from build123d import *

# Parameters (mm, degrees)
SKETCH1_W                = 285
SKETCH1_H                = 190
SKETCH1_R                = 2
SKETCH1_R_2              = 2.4
SKETCH1_R_3              = 1.75
BOSS_EXTRUDE1_DEPTH      = 3.5
SKETCH2_R                = 1.725
JETSON_HOLES_DEPTH       = 10
SKETCH3_R                = 6.35
SWITCH_HOLES_DEPTH       = 10
SKETCH5_R                = 2.25
WIRES_AND_TRACKERS_DEPTH = 10
SKETCH6_R                = 2.05
MOUNTING_HOLES_DEPTH     = 10
SKETCH7_R                = 2.05
LIDAR_MOUNT_DEPTH        = 10


with BuildPart() as part:
    # Sketch1 → Boss-Extrude1 (new body)
    with BuildSketch(Plane(origin=(0, 0, 0), x_dir=(1, 0, 0), z_dir=(0, 1, 0))):
        with Locations((142.5, 95)):
            Rectangle(SKETCH1_W, SKETCH1_H)
        with Locations(Location((67, 173, 0), (0, 0, 270))):
            Circle(SKETCH1_R, mode=Mode.SUBTRACT)
        with Locations(Location((67, 125, 0), (0, 0, 270))):
            Circle(SKETCH1_R, mode=Mode.SUBTRACT)
        with Locations(Location((119.5, 159.5, 0), (0, 0, 270))):
            Circle(SKETCH1_R, mode=Mode.SUBTRACT)
        with Locations(Location((119.5, 130.5, 0), (0, 0, 270))):
            Circle(SKETCH1_R, mode=Mode.SUBTRACT)
        with Locations(Location((215, 170, 0), (0, 0, 270))):
            Circle(SKETCH1_R_2, mode=Mode.SUBTRACT)
        with Locations(Location((268, 170, 0), (0, 0, 270))):
            Circle(SKETCH1_R_2, mode=Mode.SUBTRACT)
        with Locations(Location((268, 20, 0), (0, 0, 270))):
            Circle(SKETCH1_R_2, mode=Mode.SUBTRACT)
        with Locations(Location((215, 20, 0), (0, 0, 270))):
            Circle(SKETCH1_R_2, mode=Mode.SUBTRACT)
        with Locations(Location((210, 55, 0), (0, 0, 270))):
            Circle(SKETCH1_R_3, mode=Mode.SUBTRACT)
        with Locations(Location((165, 130, 0), (0, 0, 270))):
            Circle(SKETCH1_R_3, mode=Mode.SUBTRACT)
        with Locations(Location((210, 130, 0), (0, 0, 270))):
            Circle(SKETCH1_R_3, mode=Mode.SUBTRACT)
        with Locations(Location((165, 55, 0), (0, 0, 270))):
            Circle(SKETCH1_R_3, mode=Mode.SUBTRACT)
    extrude(amount=BOSS_EXTRUDE1_DEPTH)

    # Sketch2 → Jetson Holes (cut)
    with BuildSketch(Plane(origin=(0, 3.5, 0), x_dir=(1, 0, 0), z_dir=(0, 1, 0))):
        with Locations(Location((37, 39.5, 0), (0, 0, 270))):
            Circle(SKETCH2_R)
        with Locations(Location((37, 98, 0), (0, 0, 270))):
            Circle(SKETCH2_R)
        with Locations(Location((123.3, 98, 0), (0, 0, 270))):
            Circle(SKETCH2_R)
        with Locations(Location((123.3, 39.5, 0), (0, 0, 270))):
            Circle(SKETCH2_R)
    extrude(amount=-JETSON_HOLES_DEPTH, mode=Mode.SUBTRACT)

    # Sketch3 → switch holes (cut)
    with BuildSketch(Plane(origin=(0, 3.5, 0), x_dir=(1, 0, 0), z_dir=(0, 1, 0))):
        with Locations(Location((167.296262876, 167.817050275, 0), (0, 0, 270))):
            Circle(SKETCH3_R)
        with Locations(Location((167.296262876, 23.68564224, 0), (0, 0, 270))):
            Circle(SKETCH3_R)
    extrude(amount=-SWITCH_HOLES_DEPTH, mode=Mode.SUBTRACT)

    # Sketch5 → Wires and trackers (cut)
    with BuildSketch(Plane(origin=(0, 3.5, 0), x_dir=(1, 0, 0), z_dir=(0, 1, 0))):
        with Locations(Location((173.809093187, 44.240172362, 0), (0, 0, 270))):
            Circle(SKETCH5_R)
        with Locations(Location((9.328490985, 8.27715501, 0), (0, 0, 270))):
            Circle(SKETCH5_R)
        with Locations(Location((26.341972093, 182.045088306, 0), (0, 0, 270))):
            Circle(SKETCH5_R)
        with Locations(Location((279.649236993, 185.189806704, 0), (0, 0, 270))):
            Circle(SKETCH5_R)
        with Locations(Location((265.450893748, 120.912595142, 0), (0, 0, 270))):
            Circle(SKETCH5_R)
        with Locations(Location((279.649236993, 44.240172362, 0), (0, 0, 270))):
            Circle(SKETCH5_R)
        with Locations(Location((128.170746294, 12.293329537, 0), (0, 0, 270))):
            Circle(SKETCH5_R)
        with BuildLine():
            Line((215, 46.226982274), (265.510732016, 46.226982274))
            ThreePointArc((265.510732016, 46.226982274), (271.666947369, 40.070766921), (265.510732016, 33.914551567))
            Line((265.510732016, 33.914551567), (215, 33.914551567))
            ThreePointArc((215, 33.914551567), (208.843784647, 40.070766921), (215, 46.226982274))
        make_face()
    extrude(amount=-WIRES_AND_TRACKERS_DEPTH, mode=Mode.SUBTRACT)

    # Sketch6 → Mounting holes (cut)
    with BuildSketch(Plane(origin=(0, 3.5, 0), x_dir=(1, 0, 0), z_dir=(0, 1, 0))):
        with Locations(Location((41.27533381, 118, 0), (0, 0, 270))):
            Circle(SKETCH6_R)
        with Locations(Location((151.27533381, 118, 0), (0, 0, 270))):
            Circle(SKETCH6_R)
        with Locations(Location((230.27533381, 118, 0), (0, 0, 270))):
            Circle(SKETCH6_R)
        with Locations(Location((230.27533381, 72, 0), (0, 0, 270))):
            Circle(SKETCH6_R)
        with Locations(Location((151.27533381, 72, 0), (0, 0, 270))):
            Circle(SKETCH6_R)
        with Locations(Location((41.27533381, 72, 0), (0, 0, 270))):
            Circle(SKETCH6_R)
    extrude(amount=-MOUNTING_HOLES_DEPTH, mode=Mode.SUBTRACT)

    # Sketch7 → Lidar Mount (cut)
    with BuildSketch(Plane(origin=(0, 3.5, 0), x_dir=(1, 0, 0), z_dir=(0, 1, 0))):
        with Locations(Location((143.3, 125, 0), (0, 0, 270))):
            Circle(SKETCH7_R)
        with Locations(Location((23.3, 125, 0), (0, 0, 270))):
            Circle(SKETCH7_R)
        with Locations(Location((143.3, 65, 0), (0, 0, 270))):
            Circle(SKETCH7_R)
        with Locations(Location((23.3, 65, 0), (0, 0, 270))):
            Circle(SKETCH7_R)
    extrude(amount=-LIDAR_MOUNT_DEPTH, mode=Mode.SUBTRACT)


solid = part.part
Can you work these out from the model? Positions are in its coordinate system, mm. A direction names the side the tool comes from. Round coordinates to 2 decimals unless told otherwise and drop trailing zeros. Use a Markdown table: item, result.
1) If we mould it in two halves opening along Z, with no side actions, what happens to faces 3 (the face through (169.2, 1.77, -161.76)), 4 (the face through (141, 3.5, -96))? For each: +Z half, -Z half, draft (parallel to the pull), parting line (faces both ways), or undercut.
Geometry says:
| item | result |
|---|---|
| face 3 | undercut |
| face 4 | draft |
2) Imagine slicing it at A-A (y = 2.2). Give the number of separate pieces and of enclosed holes in the cut face, then the cut area to 3 significant figures.
Geometry says:
| item | result |
|---|---|
| separate pieces | 1 |
| enclosed holes | 36 |
| area | 52,700 mm² |
3) If I drill on line 1 along X through (y, z) = (1.2, -72); line 2 along Z through (x, y) = (123.3, 1.65) (3 decimals); line 3 along X through (y, z) = (0.7, -65), over which ranges is the centre line in solid material (lowest first)?
Geometry says:
| item | result |
|---|---|
| line 1 | x = 0 to 39.23, 43.33 to 149.23, 153.33 to 228.23, 232.33 to 285 |
| line 2 | z = -190 to -99.725, -96.275 to -41.225, -37.775 to 0 |
| line 3 | x = 0 to 21.25, 25.35 to 141.25, 145.35 to 285 |
4) On a 3-axis mill with a long thin cutter (end or side, diameter ignored), from which of +Z, -Z, +X, -X, +Y, -Y can I reach the whole of each face in a straight line? I mean faces 1 (the face through (208.845, 1.774, -39.935)), 2 (the face through (141, 0, -96)). Say none if no direction works.
Geometry says:
| item | result |
|---|---|
| face 1 | +Y, -Y |
| face 2 | +Z, -Z, +X, -X, -Y |
5) I'm going to push a flat-ended pin straight in: P1, Ø14.5, axis at x = 167.3, z = -167.82, coming from the +Y side. Where does the tip first touch, or does it pass through?
Geometry says:
| item | result |
|---|---|
| P1 | stops at y = 3.5 |
